Drawing for the job (mm, zero at the part's lowest x, y, z). A direction names the side the tool comes from. Give positions to 0.01 mm unless a question says otherwise; leave off trailing zeros. Write each loop counter-clockwise with the first axis right and the second up, starting at its lowest first coordinate (ties: lowest second). Pieces come first, ordered by that corner, then holes. Notation, with made-up numbers: (56, -29) - (110, -29) arc R17 cw to (110, 2) - close; hole circle Ø4 at (6, 1). An arc over 180 degrees is marked (long way). Write item = value, one per line. Start each with the question number.
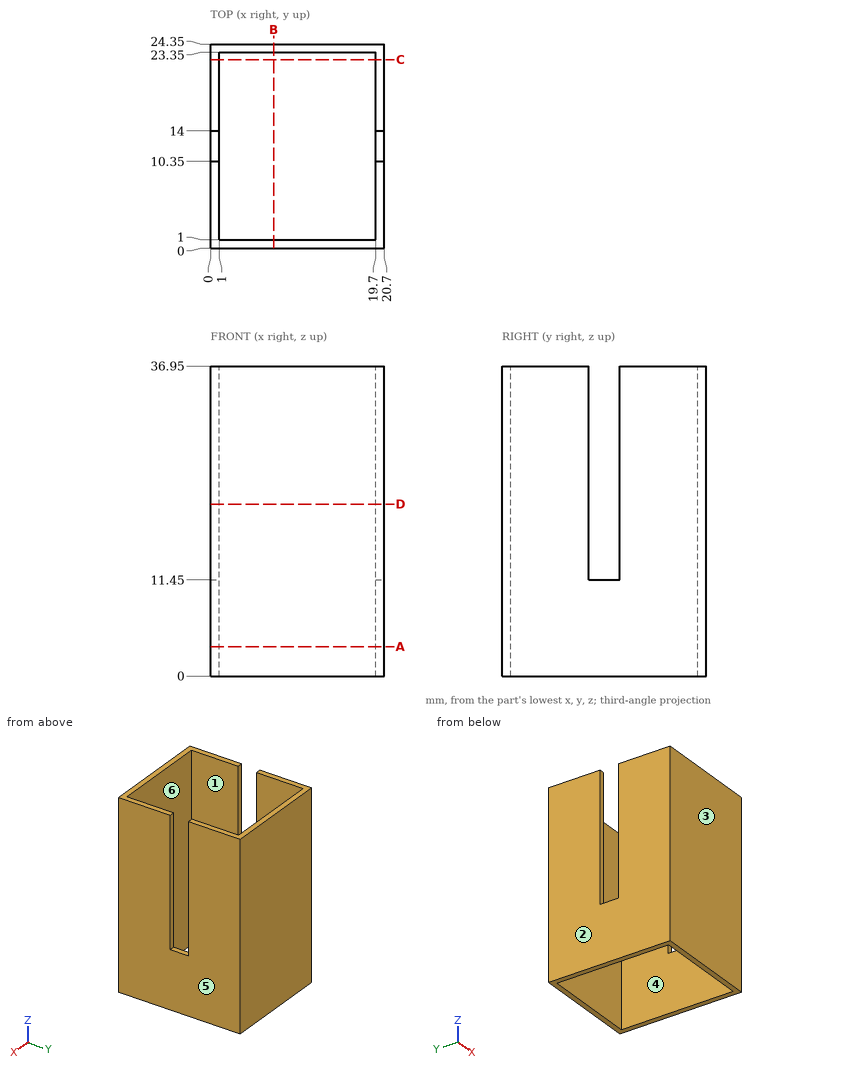
1. Pin check, flat tips, straight feed: pin 1 Ø4 at (x, y) = (16, 21.5) entering from +Z; pin 2 Ø0.5 at (x, y) = (0.5, 13) entering from +Z. Stop position of each tip, or through.
2. Cut at A-A (z = 3.5). Give the cut face in (x, y), then the cut area to 3 significant figures.
3. Cut at B-B (x = 7.5). Give the cut face in (y, z).
4. Cut at C-C (y = 22.5). Give the cut face in (x, z), then the cut area to 3 significant figures.
5. Wall check: line 1 along Y through (x, z) = (13, 11.5); line 2 along Y through (x, z) = (20.25, 29); line 3 along X through (y, z) = (5.75, 10.5). Give the ranges that are in metal, low to high.
6. Tool access for the marked faces 5 and 6: list every direction of +Z, -Z, +X, -X, +Y, -Y with a clear straight run to the whole face (end or side of a thin tool).
7. Mould opens along Y. For the marked faces 1, 2, 3 and 4 say: +Y half, -Y half, draft (parallel to the pull), parting line (faces both ways), or undercut.
8. Cut at D-D (z = 20.5). Give the cut face in (x, y).
Output:
q1.pin_1 = 36.95
q1.pin_2 = 11.45
q2.outline = (0, 0) - (20.7, 0) - (20.7, 24.35) - (0, 24.35) - close; hole (1, 1) - (19.7, 1) - (19.7, 23.35) - (1, 23.35) - close
q2.area = 86.1 mm2
q3.outline = (0, 0) - (1, 0) - (1, 36.95) - (0, 36.95) - close; (23.35, 0) - (24.35, 0) - (24.35, 36.95) - (23.35, 36.95) - close
q4.outline = (0, 0) - (1, 0) - (1, 36.95) - (0, 36.95) - close; (19.7, 0) - (20.7, 0) - (20.7, 36.95) - (19.7, 36.95) - close
q4.area = 73.9 mm2
q5.line_1 = 0 to 1, 23.35 to 24.35
q5.line_2 = 0 to 10.35, 14 to 24.35
q5.line_3 = 0 to 1, 19.7 to 20.7
q6.face_5 = +Z, -Z, +X, +Y, -Y
q6.face_6 = +Z, -Z
q7.face_1 = undercut
q7.face_2 = draft
q7.face_3 = -Y half
q7.face_4 = undercut
q8.outline = (0, 0) - (20.7, 0) - (20.7, 10.35) - (19.7, 10.35) - (19.7, 1) - (1, 1) - (1, 10.35) - (0, 10.35) - close; (0, 14) - (1, 14) - (1, 23.35) - (19.7, 23.35) - (19.7, 14) - (20.7, 14) - (20.7, 24.35) - (0, 24.35) - close
